```python
from build123d import *

# Parameters (mm, degrees)
SKETCH1_W           = 20
SKETCH1_H           = 60
BOSS_EXTRUDE1_DEPTH = 6
SKETCH2_R           = 1.5
CUT_EXTRUDE1_DEPTH  = 10


with BuildPart() as part:
    # Sketch1 → Boss-Extrude1 (new body)
    with BuildSketch(Plane.XY):
        Rectangle(SKETCH1_W, SKETCH1_H)
    extrude(amount=BOSS_EXTRUDE1_DEPTH)

    # Sketch2 → Cut-Extrude1 (cut)
    with BuildSketch(Plane(origin=(0, 30, 0), x_dir=(1, 0, 0), z_dir=(0, 1, 0))):
        with Locations((0, -3)):
            Circle(SKETCH2_R)
    cut_extrude1 = extrude(amount=-CUT_EXTRUDE1_DEPTH, mode=Mode.SUBTRACT)

    # Mirror1: Cut-Extrude1 across plane
    add(cut_extrude1.mirror(Plane.ZX), mode=Mode.SUBTRACT)


solid = part.part
```
Verification items for the finished model (mm, model axes). A direction names the side the tool comes from. Give positions to 0.01 mm unless a question says otherwise; leave off trailing zeros. Order: outer loops, then holes, each group sorted by start corner. A loop starts at its lowest first (then second) coordinate and runs counter-clockwise, first axis right, second up. Notation, with made-up numbers: (-25.75, 66) -> (-9.75, 66) arc R27 ccw to (-9.75, 93) -> close; hole circle Ø2 at (-18.5, -37.75). An arc over 180 degrees is marked (long way). One line per item, written item: value.
(1) Tool access check on faces 1 (the face through (0, -20, 3)), 2 (the face through (-10, 0, 3)), 3 (the face through (-0.195, 25.07, 1.513)). Record the directions out of +Z, -Z, +X, -X, +Y, -Y that give a thin tool (end or side, any length) a straight path to the whole face; none if there is none.
Final values:
face 1: -Y
face 2: +Z, -Z, -X, +Y, -Y
face 3: +Y
(2) Gauge pin test, flat end, axial feed: pin 1 (2.5 mm diameter, centred on x = 0, z = 3, fed in from -Y). Record the tip position at first contact, or that the pin passes through.
Final values:
pin 1: y = -20
(3) Scan lines: line 1 along X through (y, z) = (-27.25, 3); line 2 along Z through (x, y) = (0, 24.75); line 3 along X through (y, z) = (-23.5, 1.65). Record each from-to range of solid material in increasing order. Write a range as [from, to].
Final values:
line 1: [-10, -1.5], [1.5, 10]
line 2: [0, 1.5], [4.5, 6]
line 3: [-10, -0.65], [0.65, 10]
(4) Sectioned sample at B-B on x = 0. Record the cut outline in (y, z), then the cut area to 3 significant figures.
Final values:
outline: (-30, 0) -> (30, 0) -> (30, 1.5) -> (20, 1.5) -> (20, 4.5) -> (30, 4.5) -> (30, 6) -> (-30, 6) -> (-30, 4.5) -> (-20, 4.5) -> (-20, 1.5) -> (-30, 1.5) -> close
area: 300 mm^2
(5) Sectioned sample at A-A on y = -22. Record the cut outline in (x, z), then the cut area to 3 significant figures.
Final values:
outline: (-10, 0) -> (10, 0) -> (10, 6) -> (-10, 6) -> close; hole circle Ø3 at (0, 3)
area: 113 mm^2
(6) Draft check along Z on faces 4 (the face through (0, 0, 0)), 5 (the face through (0, 20, 3)), 6 (the face through (10, 0, 3)). Enter one of: pulls with the +Z half, pulls with the -Z half, needs draft (parallel to the pull), parting line crosses it, or undercut.
Final values:
face 4: pulls with the -Z half
face 5: undercut
face 6: needs draft
(7) Sectioned sample at C-C on z = 3. Record the cut outline in (x, y), then the cut area to 3 significant figures.
Final values:
outline: (-10, -30) -> (-1.5, -30) -> (-1.5, -20) -> (1.5, -20) -> (1.5, -30) -> (10, -30) -> (10, 30) -> (1.5, 30) -> (1.5, 20) -> (-1.5, 20) -> (-1.5, 30) -> (-10, 30) -> close
area: 1,140 mm^2
